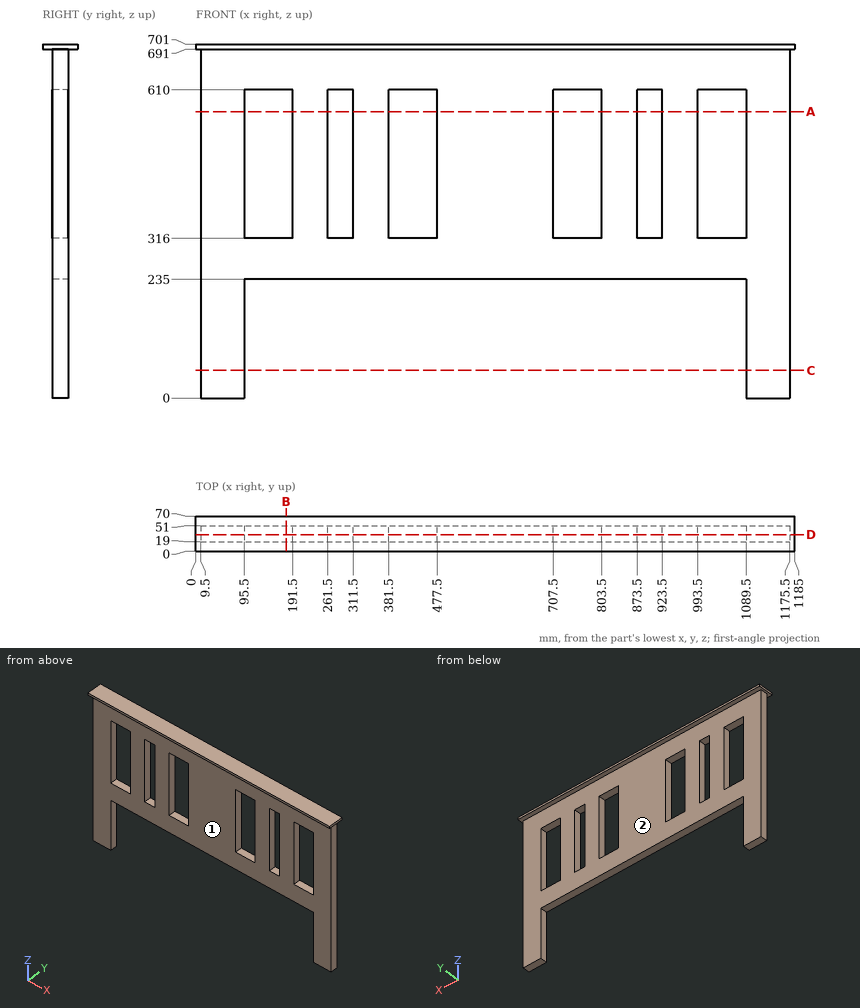
Source: three-view drawing plus pictorial views. Frame: mm from the lowest corner of the part. A direction names the side the tool comes from. Give positions to 0.01 mm unless a question says otherwise; leave off trailing zeros. Order: outer loops, then holes, each group sorted by start corner. A loop starts at its lowest first (then second) coordinate and runs counter-clockwise, first axis right, second up. Notation, with made-up numbers: (31, 39.25) - (71, 39.25) arc R24 ccw to (71, 56.25) - close; hole circle Ø6 at (-18, 6). An arc over 180 degrees is marked (long way). Answer as a JSON object with one key per item and string values. Group by question number.
Q1. Cut plane B-B, the plane x = 178.5. Output: boundary loops of the cut face in (y, z), then the cut area to 3 significant figures.
Q2. Set-up query: the marked faces 1 and 2. Return all of +Z, -Z, +X, -X, +Y, -Y with unobstructed straight access to the full face (end or side cutting, diameter ignored); none if empty.
Q3. Line query: probe 1 along Z at (x, y) = (114, 36.5); probe 2 along X at (y, z) = (45.5, 120); probe 3 along Y at (x, z) = (705, 414). Output: solid intervals per line, ascending.
Q4. First-contact query: pin 1 Ø9.5 at (y, z) = (33, 531) entering from -X; pin 2 Ø4 at (y, z) = (40, 443) entering from +X; pin 3 Ø8 at (x, y) = (579.5, 58.5) entering from -Z. Flat tips, straight axial feed; report the tip coordinate or a pass-through.
Q5. Cut plane D-D, the plane y = 33.5. Count the separate pieces of the cut face and the enclosed holes in it, then the cut area to 3 significant figures.
Q6. Cut plane C-C, the plane z = 55. Output: boundary loops of the cut face in (x, y).
Q7. Cut plane A-A, the plane z = 567. Output: boundary loops of the cut face in (x, y), then the cut area to 3 significant figures.
Results:
{
 "1": {"outline": "(0, 691) - (19, 691) - (19, 610) - (51, 610) - (51, 691) - (70, 691) - (70, 701) - (0, 701) - close; (19, 235) - (51, 235) - (51, 316) - (19, 316) - close", "area": "5,880 mm^2"},
 "2": {"face 1": "-Z, +X, -X, -Y", "face 2": "-Z, +X, -X, +Y"},
 "3": {"probe 1": "235 to 316, 610 to 701", "probe 2": "9.5 to 95.5, 1089.5 to 1175.5", "probe 3": "19 to 51"},
 "4": {"pin 1": "x = 9.5", "pin 2": "x = 1175.5", "pin 3": "z = 691"},
 "5": {"separate pieces": "1", "enclosed holes": "6", "area": "442,000 mm^2"},
 "6": {"outline": "(9.5, 19) - (95.5, 19) - (95.5, 51) - (9.5, 51) - close; (1089.5, 19) - (1175.5, 19) - (1175.5, 51) - (1089.5, 51) - close"},
 "7": {"outline": "(9.5, 19) - (95.5, 19) - (95.5, 51) - (9.5, 51) - close; (191.5, 19) - (261.5, 19) - (261.5, 51) - (191.5, 51) - close; (311.5, 19) - (381.5, 19) - (381.5, 51) - (311.5, 51) - close; (477.5, 19) - (707.5, 19) - (707.5, 51) - (477.5, 51) - close; (803.5, 19) - (873.5, 19) - (873.5, 51) - (803.5, 51) - close; (923.5, 19) - (993.5, 19) - (993.5, 51) - (923.5, 51) - close; (1089.5, 19) - (1175.5, 19) - (1175.5, 51) - (1089.5, 51) - close", "area": "21,800 mm^2"}
}
